from build123d import *

# Parameters (mm, degrees)
BOSS_EXTRUDE1_DEPTH = 3.175
BOSS_EXTRUDE2_DEPTH = 3.175
SKETCH3_W           = 6.236959702
SKETCH3_H           = 41.352711554
BOSS_EXTRUDE3_DEPTH = 3.175
SKETCH4_R           = 1.27
BOSS_EXTRUDE4_DEPTH = 3.175
BOSS_EXTRUDE5_REACH = 20.766
SKETCH6_W           = 1.202138058
SKETCH6_H           = 43.066281197
CUT_EXTRUDE1_REACH  = 11.525


with BuildPart() as part:
    # Sketch1 → Boss-Extrude1 (new body)
    with BuildSketch(Plane.XY):
        with BuildLine():
            Line((-17.114253333, -23.707583903), (-17.114253333, 23.707583903))
            ThreePointArc((-17.114253333, 23.707583903), (0, 30.782200079), (17.114253333, 23.707583903))
            Line((17.114253333, 23.707583903), (17.114253333, -23.707583903))
            ThreePointArc((17.114253333, -23.707583903), (0, -19.732802645), (-17.114253333, -23.707583903))
        make_face()
    extrude(amount=BOSS_EXTRUDE1_DEPTH)

    # Sketch2 → Boss-Extrude2 (add)
    with BuildSketch(Plane(origin=(0, 0, 0), x_dir=(-1, 0, 0), z_dir=(0, 0, -1))):
        with BuildLine():
            Line((-1.65128862, -19.767928257), (-1.65128862, 22.268343179))
            Line((-1.65128862, 22.268343179), (-1.65128862, 23.29835294))
            Line((-1.65128862, 23.29835294), (-2.853426735, 23.29835294))
            Line((-2.853426735, 23.29835294), (-2.853426735, -19.837781624))
            ThreePointArc((-2.853426735, -19.837781624), (-2.25262846, -19.798194915), (-1.65128862, -19.767928257))
        make_face()
        with BuildLine():
            Line((1.65128862, 23.29835294), (1.65128862, 22.268343179))
            Line((1.65128862, 22.268343179), (1.65128862, -19.767928257))
            ThreePointArc((1.65128862, -19.767928257), (2.25262846, -19.798194915), (2.853426735, -19.837781624))
            Line((2.853426735, -19.837781624), (2.853426735, 23.29835294))
            Line((2.853426735, 23.29835294), (1.65128862, 23.29835294))
        make_face()
    extrude(amount=BOSS_EXTRUDE2_DEPTH)

    # Sketch3 → Boss-Extrude3 (add)
    with BuildSketch(Plane.XY.offset(3.175)):
        with Locations((0, -20.33746726)):
            Rectangle(SKETCH3_W, SKETCH3_H)
    extrude(amount=-BOSS_EXTRUDE3_DEPTH)

    # Sketch4 → Boss-Extrude4 (add)
    with BuildSketch(Plane.XY.offset(3.175)):
        with Locations((0, -31.201683403)):
            Circle(SKETCH4_R)
    extrude(amount=BOSS_EXTRUDE4_DEPTH)

    # Sketch6 → Boss-Extrude5 (add, up to next)
    with BuildSketch(Plane.ZY.offset(-1.65128862), mode=Mode.PRIVATE) as boss_extrude5_sk1:
        with Locations((-2.573930971, 1.765212341)):
            Rectangle(SKETCH6_W, SKETCH6_H)
    boss_extrude5_tool1 = extrude(boss_extrude5_sk1.sketch, amount=BOSS_EXTRUDE5_REACH, mode=Mode.PRIVATE) - part.part
    add(boss_extrude5_tool1.solids().sort_by_distance((1.651289, 1.765212, -2.573931))[0])

    # Sketch8 → Cut-Extrude1 (cut, up to next)
    with BuildSketch(Plane(origin=(0, 0, -3.175), x_dir=(-1, 0, 0), z_dir=(0, 0, -1)), mode=Mode.PRIVATE) as cut_extrude1_sk1:
        Polygon((0, 23.29835294), (-0.889, 23.29835294), (-0.889, -19.767928257), (0.889, -19.767928257), (0.889, 23.29835294), align=None)
    cut_extrude1_tool1 = extrude(cut_extrude1_sk1.sketch, amount=-CUT_EXTRUDE1_REACH, mode=Mode.PRIVATE) & part.part
    add(cut_extrude1_tool1.solids().sort_by_distance((0, 1.765212, -3.175))[0], mode=Mode.SUBTRACT)


solid = part.part
Check sheet for the modelled part. Datum: model origin and axes. Units: mm. A direction names the side the tool comes from. Give positions to 0.01 mm unless a question says otherwise; leave off trailing zeros. Order: outer loops, then holes, each group sorted by start corner. A loop starts at its lowest first (then second) coordinate and runs counter-clockwise, first axis right, second up. Notation, with made-up numbers: M 77,42.5 L 92,42.5 A12 cw 92,60.5 Z; hole C 45,89 d6. An arc over 180 degrees is marked long. Answer as CSV lines item,"result". Start each with the question number.
Item 1: Thickness scan on line 1 (X direction, y = -5.5, z = -2.5); line 2 (X direction, y = -19.5, z = -1); line 3 (Z direction, x = -11.5, y = -4) (3 decimals). Record the ranges inside material, lowest first. Write a range as [from, to].
Item 2: Cross-section at D-D on z = 4.5. Enter the section's corners in (x, y), plus the area to 3 significant figures.
Item 3: Tool access check on faces 1 (the face through (0.889, 2, -3)), 2 (the face through (-2.853, 1, -2)), 3 (the face through (3.118, -31, 2)), 4 (the face through (-2.244, -19.798, -1.565)). Record the directions out of +Z, -Z, +X, -X, +Y, -Y that give a thin tool (end or side, any length) a straight path to the whole face; none if there is none.
Item 4: Cross-section at C-C on z = 1.5. Enter the section's corners in (x, y), plus the area to 3 significant figures.
Item 5: Gauge pin test, flat ends, axial feed: P1, Ø1, axis at y = -25, z = 1, coming from the +X side; P2, Ø0.6, axis at x = -1.5, z = -3, coming from the -Y side; P3, Ø2.5, axis at y = -25.5, z = 2, coming from the -X side. Record the tip position at first contact, or that the pin passes through.
Item 6: Mould release check, pull along Z, two halves, no side actions. Record for faces 5 (the face through (0, -31, 6.35)), 6 (the face through (-1.651, 2, -1)), 7 (the face through (-17.114, 0, 2)): +Z half, -Z half, draft (parallel to the pull), parting line (faces both ways), or undercut.
Item 7: Cross-section at A-A on y = 20. Enter the section's corners in (x, z) (3 decimals).
Item 8: Cross-section at B-B on x = 0. Enter the section's corners in (y, z) (3 decimals), plus the area to 3 significant figures.
Established:
1,line 1,"x = [-2.85, -0.89], [0.89, 2.85]"
1,line 2,"x = [-2.85, -1.65], [1.65, 2.85]"
1,line 3,"z = [0, 3.175]"
2,outline,"C 0,-31.2 d2.54"
2,area,"5.07 mm^2"
3,face 1,"-Z, +Y, -Y"
3,face 2,"-Z, -X, +Y, -Y"
3,face 3,"+Z, -Z, -Y"
3,face 4,"-Z, -Y"
4,outline,"M -17.11,-23.71 A38.83 cw -3.12,-19.86 L -3.12,-41.01 L 3.12,-41.01 L 3.12,-19.86 A38.83 cw 17.11,-23.71 L 17.11,23.71 A24.24 ccw -17.11,23.71 Z"
4,area,"1,830 mm^2"
5,P1,"stops at x = 3.12"
5,P2,"stops at y = -19.77"
5,P3,"stops at x = -3.12"
6,face 5,"+Z half"
6,face 6,"undercut"
6,face 7,"draft"
7,outline,"M -17.114,0 L -2.853,0 L -2.853,-3.175 L -0.889,-3.175 L -0.889,-1.973 L -1.651,-1.973 L -1.651,0 L 1.651,0 L 1.651,-1.973 L 0.889,-1.973 L 0.889,-3.175 L 2.853,-3.175 L 2.853,0 L 17.114,0 L 17.114,3.175 L -17.114,3.175 Z"
8,outline,"M -41.014,0 L 30.782,0 L 30.782,3.175 L -29.932,3.175 L -29.932,6.35 L -32.472,6.35 L -32.472,3.175 L -41.014,3.175 Z"
8,area,"236 mm^2"
